from build123d import *

# Parameters (mm, degrees)
F0_R     = 1.9939
F1_DEPTH = 5.9436


with BuildPart() as f1:
    # F0 (on Top) → F1 (new body)
    with BuildSketch(Plane.XY):
        with BuildLine():
            ThreePointArc((1.165337, 3.64131), (1.103355, 3.575271), (1.013135, 3.567322))
            ThreePointArc((1.013135, 3.567322), (0.825197, 3.615423), (0.635, 3.653629))
            ThreePointArc((0.635, 3.653629), (0.557163, 3.699936), (0.529973, 3.786328))
            ThreePointArc((0.529973, 3.786328), (0.474446, 4.2945), (0.254, 4.755722))
            ThreePointArc((0.254, 4.755722), (0, 4.7625), (-0.254, 4.755722))
            ThreePointArc((-0.254, 4.755722), (-0.474446, 4.2945), (-0.529973, 3.786328))
            ThreePointArc((-0.529973, 3.786328), (-0.557163, 3.699936), (-0.635, 3.653629))
            ThreePointArc((-0.635, 3.653629), (-0.825197, 3.615423), (-1.013135, 3.567322))
            ThreePointArc((-1.013135, 3.567322), (-1.103355, 3.575271), (-1.165337, 3.64131))
            ThreePointArc((-1.165337, 3.64131), (-1.435853, 4.075065), (-1.834584, 4.394964))
            ThreePointArc((-1.834584, 4.394964), (-2.066371, 4.290864), (-2.292276, 4.174551))
            ThreePointArc((-2.292276, 4.174551), (-2.290774, 3.663356), (-2.120315, 3.181417))
            ThreePointArc((-2.120315, 3.181417), (-2.107329, 3.091783), (-2.157365, 3.01629))
            ThreePointArc((-2.157365, 3.01629), (-2.31215, 2.899344), (-2.460606, 2.774463))
            ThreePointArc((-2.460606, 2.774463), (-2.545341, 2.74248), (-2.629838, 2.775086))
            ThreePointArc((-2.629838, 2.775086), (-3.061763, 3.048513), (-3.559807, 3.163729))
            ThreePointArc((-3.559807, 3.163729), (-3.723472, 2.96937), (-3.876539, 2.766559))
            ThreePointArc((-3.876539, 2.766559), (-3.653387, 2.30664), (-3.290703, 1.946387))
            ThreePointArc((-3.290703, 1.946387), (-3.240112, 1.871264), (-3.252438, 1.781537))
            ThreePointArc((-3.252438, 1.781537), (-3.341153, 1.609014), (-3.420724, 1.432088))
            ThreePointArc((-3.420724, 1.432088), (-3.48319, 1.366507), (-3.573466, 1.359222))
            ThreePointArc((-3.573466, 1.359222), (-4.081254, 1.418166), (-4.579966, 1.305879))
            ThreePointArc((-4.579966, 1.305879), (-4.643094, 1.059756), (-4.693006, 0.810616))
            ThreePointArc((-4.693006, 0.810616), (-4.292402, 0.493066), (-3.809327, 0.325852))
            ThreePointArc((-3.809327, 0.325852), (-3.731151, 0.280119), (-3.703326, 0.19393))
            ThreePointArc((-3.703326, 0.19393), (-3.7084, 0), (-3.703326, -0.19393))
            ThreePointArc((-3.703326, -0.19393), (-3.731151, -0.280119), (-3.809327, -0.325852))
            ThreePointArc((-3.809327, -0.325852), (-4.292402, -0.493066), (-4.693006, -0.810616))
            ThreePointArc((-4.693006, -0.810616), (-4.643094, -1.059756), (-4.579966, -1.305879))
            ThreePointArc((-4.579966, -1.305879), (-4.081254, -1.418166), (-3.573466, -1.359222))
            ThreePointArc((-3.573466, -1.359222), (-3.48319, -1.366507), (-3.420724, -1.432088))
            ThreePointArc((-3.420724, -1.432088), (-3.341153, -1.609014), (-3.252438, -1.781537))
            ThreePointArc((-3.252438, -1.781537), (-3.240112, -1.871264), (-3.290703, -1.946387))
            ThreePointArc((-3.290703, -1.946387), (-3.653387, -2.30664), (-3.876539, -2.766559))
            ThreePointArc((-3.876539, -2.766559), (-3.723472, -2.96937), (-3.559807, -3.163729))
            ThreePointArc((-3.559807, -3.163729), (-3.061763, -3.048513), (-2.629838, -2.775086))
            ThreePointArc((-2.629838, -2.775086), (-2.545341, -2.74248), (-2.460606, -2.774463))
            ThreePointArc((-2.460606, -2.774463), (-2.31215, -2.899344), (-2.157365, -3.01629))
            ThreePointArc((-2.157365, -3.01629), (-2.107329, -3.091783), (-2.120315, -3.181417))
            ThreePointArc((-2.120315, -3.181417), (-2.290774, -3.663356), (-2.292276, -4.174551))
            ThreePointArc((-2.292276, -4.174551), (-2.066371, -4.290864), (-1.834584, -4.394964))
            ThreePointArc((-1.834584, -4.394964), (-1.435853, -4.075065), (-1.165337, -3.64131))
            ThreePointArc((-1.165337, -3.64131), (-1.103355, -3.575271), (-1.013135, -3.567322))
            ThreePointArc((-1.013135, -3.567322), (-0.825197, -3.615423), (-0.635, -3.653629))
            ThreePointArc((-0.635, -3.653629), (-0.557163, -3.699936), (-0.529973, -3.786328))
            ThreePointArc((-0.529973, -3.786328), (-0.474446, -4.2945), (-0.254, -4.755722))
            ThreePointArc((-0.254, -4.755722), (0, -4.7625), (0.254, -4.755722))
            ThreePointArc((0.254, -4.755722), (0.474446, -4.2945), (0.529973, -3.786328))
            ThreePointArc((0.529973, -3.786328), (0.557163, -3.699936), (0.635, -3.653629))
            ThreePointArc((0.635, -3.653629), (0.825197, -3.615423), (1.013135, -3.567322))
            ThreePointArc((1.013135, -3.567322), (1.103355, -3.575271), (1.165337, -3.64131))
            ThreePointArc((1.165337, -3.64131), (1.435853, -4.075065), (1.834584, -4.394964))
            ThreePointArc((1.834584, -4.394964), (2.066371, -4.290864), (2.292276, -4.174551))
            ThreePointArc((2.292276, -4.174551), (2.290774, -3.663356), (2.120315, -3.181417))
            ThreePointArc((2.120315, -3.181417), (2.107329, -3.091783), (2.157365, -3.01629))
            ThreePointArc((2.157365, -3.01629), (2.31215, -2.899344), (2.460606, -2.774463))
            ThreePointArc((2.460606, -2.774463), (2.545341, -2.74248), (2.629838, -2.775086))
            ThreePointArc((2.629838, -2.775086), (3.061763, -3.048513), (3.559807, -3.163729))
            ThreePointArc((3.559807, -3.163729), (3.723472, -2.96937), (3.876539, -2.766559))
            ThreePointArc((3.876539, -2.766559), (3.653387, -2.30664), (3.290703, -1.946387))
            ThreePointArc((3.290703, -1.946387), (3.240112, -1.871264), (3.252438, -1.781537))
            ThreePointArc((3.252438, -1.781537), (3.341153, -1.609014), (3.420724, -1.432088))
            ThreePointArc((3.420724, -1.432088), (3.48319, -1.366507), (3.573466, -1.359222))
            ThreePointArc((3.573466, -1.359222), (4.081254, -1.418166), (4.579966, -1.305879))
            ThreePointArc((4.579966, -1.305879), (4.643094, -1.059756), (4.693006, -0.810616))
            ThreePointArc((4.693006, -0.810616), (4.292402, -0.493066), (3.809327, -0.325852))
            ThreePointArc((3.809327, -0.325852), (3.731151, -0.280119), (3.703326, -0.19393))
            ThreePointArc((3.703326, -0.19393), (3.7084, 0), (3.703326, 0.19393))
            ThreePointArc((3.703326, 0.19393), (3.731151, 0.280119), (3.809327, 0.325852))
            ThreePointArc((3.809327, 0.325852), (4.292402, 0.493066), (4.693006, 0.810616))
            ThreePointArc((4.693006, 0.810616), (4.643094, 1.059756), (4.579966, 1.305879))
            ThreePointArc((4.579966, 1.305879), (4.081254, 1.418166), (3.573466, 1.359222))
            ThreePointArc((3.573466, 1.359222), (3.48319, 1.366507), (3.420724, 1.432088))
            ThreePointArc((3.420724, 1.432088), (3.341153, 1.609014), (3.252438, 1.781537))
            ThreePointArc((3.252438, 1.781537), (3.240112, 1.871264), (3.290703, 1.946387))
            ThreePointArc((3.290703, 1.946387), (3.653387, 2.30664), (3.876539, 2.766559))
            ThreePointArc((3.876539, 2.766559), (3.723472, 2.96937), (3.559807, 3.163729))
            ThreePointArc((3.559807, 3.163729), (3.061763, 3.048513), (2.629838, 2.775086))
            ThreePointArc((2.629838, 2.775086), (2.545341, 2.74248), (2.460606, 2.774463))
            ThreePointArc((2.460606, 2.774463), (2.31215, 2.899344), (2.157365, 3.01629))
            ThreePointArc((2.157365, 3.01629), (2.107329, 3.091783), (2.120315, 3.181417))
            ThreePointArc((2.120315, 3.181417), (2.290774, 3.663356), (2.292276, 4.174551))
            ThreePointArc((2.292276, 4.174551), (2.066371, 4.290864), (1.834584, 4.394964))
            ThreePointArc((1.834584, 4.394964), (1.435853, 4.075065), (1.165337, 3.64131))
        make_face()
        Circle(F0_R, mode=Mode.SUBTRACT)
    extrude(amount=F1_DEPTH)


solid = f1.part
Work out the finished part from the listing and answer in its coordinate system (mm). A direction names the side the tool comes from. Give positions to 0.01 mm unless a question says otherwise; leave off trailing zeros. Order: outer loops, then holes, each group sorted by start corner. A loop starts at its lowest first (then second) coordinate and runs counter-clockwise, first axis right, second up. Notation, with made-up numbers: (27.5, 4.5) -> (86.5, 4.5) arc R14 cw to (86.5, 16.5) -> close; hole circle Ø4 at (89, 37). An arc over 180 degrees is marked (long way). One line per item, written item: value.
Item 1: Determine the mould class of faces 5 (the flat face through (-0.1, 2.2, 5.944)), 6 (the cylindrical face through (4.299, -0.497, 2.93)), 7 (the cylindrical face through (-4.088, -1.418, 2.93)), 8 (the cylindrical face through (-3.658, 2.313, 2.93)) for opening direction X: released by +X, released by -X, zero draft, split by the parting line, or undercut.
Answer sheet:
face 5: zero draft
face 6: released by +X
face 7: undercut
face 8: released by -X
Item 2: Find section A-A, the plane x = 0. Give the vertices of the cut face in (y, z), plus the area to 3 significant figures.
Answer sheet:
outline: (-4.76, 0) -> (-1.99, 0) -> (-1.99, 5.94) -> (-4.76, 5.94) -> close; (1.99, 0) -> (4.76, 0) -> (4.76, 5.94) -> (1.99, 5.94) -> close
area: 32.9 mm²
Item 3: A tool of negligible diameter and unlimited length cuts with its end or side. For faces 1 (the cylindrical face through (-2.29, -3.66, 2.93)), 2 (the cylindrical face through (3.055, -3.046, 2.93)), 3 (the cylindrical face through (3.07, 3.05, 2.93)), 4 (the cylindrical face through (-4.07, 1.42, 2.93)), from which of +Z, -Z, +X, -X, +Y, -Y can it reach the whole face along a straight path? Write none if from no direction.
Answer sheet:
face 1: +Z, -Z, -X
face 2: +Z, -Z, -Y
face 3: +Z, -Z, +Y
face 4: +Z, -Z
Item 4: Flat-ended cylindrical pins translate along their axes: P1, Ø3, axis at y = 3.5, z = 2.5, coming from the +X side; P2, Ø1, axis at x = -2.5, z = 1.5, coming from the +Y side; P3, Ø1, axis at x = 3, z = 3, coming from the +Y side. Find the tip coordinate at first contact, or state that the pin passes through.
Answer sheet:
P1: x = 3.88
P2: y = 4.32
P3: y = 3.16
Item 5: Find section B-B, the plane y = 0. Give the vertices of the cut face in (x, z).
Answer sheet:
outline: (-3.71, 0) -> (-1.99, 0) -> (-1.99, 5.94) -> (-3.71, 5.94) -> close; (1.99, 0) -> (3.71, 0) -> (3.71, 5.94) -> (1.99, 5.94) -> close
Item 6: Straight lines are drawn through the part: probe 1 along X at (y, z) = (-4, 5.2); probe 2 along Y at (x, z) = (-3.5, 5.65); probe 3 along Y at (x, z) = (0, 4.2). For each, find the intervals that lie inside material, in ascending order.
Answer sheet:
probe 1: -2.31 to -1.37, -0.53 to 0.53, 1.37 to 2.31
probe 2: -3.16 to -2.12, -1.36 to 1.36, 2.12 to 3.16
probe 3: -4.76 to -1.99, 1.99 to 4.76
